from build123d import *

# Parameters (mm, degrees)
ESQUISSE1_W             = 39.8
ESQUISSE1_H             = 4.9
BOSS_EXTRU_1_DEPTH      = 5
ENL_V_MAT_EXTRU_1_REACH = 7
BOSS_EXTRU_2_DEPTH      = 5


with BuildPart() as part:
    # Esquisse1 → Boss.-Extru.1 (new body)
    with BuildSketch(Plane.XY):
        Polygon((100.1, 330.041421356), (128.425692604, 301.715728753), (124.890158698, 298.180194847), (153.033008589, 270.037344955), (156.568542495, 273.572878861), (200.043297184, 230.098124172), (196.507763279, 226.562590266), (211.415404008, 211.654949536), (214.950937914, 215.190483442), (230.1, 200.041421356), (230.1, 159.9), (225.1, 159.9), (225.1, 120.1), (230.1, 120.1), (230.1, 79.9), (225.1, 79.9), (225.1, 40.1), (230.1, 40.1), (230.1, -0.1), (-0.1, -0.1), (-0.1, 50.1), (4.9, 50.1), (4.9, 99.9), (-0.1, 99.9), (-0.1, 150.1), (4.9, 150.1), (4.9, 199.9), (-0.1, 199.9), (-0.1, 250.1), (4.9, 250.1), (4.9, 299.9), (-0.1, 299.9), (-0.1, 350.1), (4.9, 350.1), (4.9, 399.9), (-0.1, 399.9), (-0.1, 450.1), (4.9, 450.1), (4.9, 499.9), (-0.1, 499.9), (-0.1, 550.1), (4.9, 550.1), (4.9, 599.9), (-0.1, 599.9), (-0.1, 650.1), (4.9, 650.1), (4.9, 699.9), (-0.1, 699.9), (-0.1, 750.1), (60.1, 750.1), (60.1, 745.1), (74.9, 745.1), (74.9, 750.1), (100.1, 750.1), (100.1, 699.9), (95.1, 699.9), (95.1, 650.1), (100.1, 650.1), (100.1, 599.9), (95.1, 599.9), (95.1, 550.1), (100.1, 550.1), (100.1, 499.9), (95.1, 499.9), (95.1, 450.1), (100.1, 450.1), (100.1, 399.9), (95.1, 399.9), (95.1, 350.1), (100.1, 350.1), align=None)
        with Locations((145, 232.55)):
            Rectangle(ESQUISSE1_W, ESQUISSE1_H, mode=Mode.SUBTRACT)
    extrude(amount=BOSS_EXTRU_1_DEPTH)

    # Esquisse3 → Enlèv. mat.-Extru.1 (cut, up to next)
    with BuildSketch(Plane.XY.offset(5), mode=Mode.PRIVATE) as enl_v_mat_extru_1_sk1:
        with BuildLine():
            Line((225.1, 156.548997307), (230.1, 156.548997307))
            Line((230.1, 156.548997307), (230.1, 200.041421356))
            Line((230.1, 200.041421356), (185.204076401, 244.937344955))
            Line((185.204076401, 244.937344955), (181.668542495, 241.401811049))
            Line((181.668542495, 241.401811049), (195.810678119, 227.259675426))
            ThreePointArc((195.810678119, 227.259675426), (217.487953251, 194.817340544), (225.1, 156.548997307))
        make_face()
    enl_v_mat_extru_1_tool1 = extrude(enl_v_mat_extru_1_sk1.sketch, amount=-ENL_V_MAT_EXTRU_1_REACH, mode=Mode.PRIVATE) & part.part
    add(enl_v_mat_extru_1_tool1.solids().sort_by_distance((215.811514, 201.214449, 5))[0], mode=Mode.SUBTRACT)

    # Esquisse4 → Boss.-Extru.2 (add)
    with BuildSketch(Plane.XY.offset(5)):
        with BuildLine():
            Line((100.1, 350.1), (100.1, 330.041421356))
            Line((100.1, 330.041421356), (114.28355698, 315.857864376))
            ThreePointArc((114.28355698, 315.857864376), (103.786186359, 331.56828974), (100.1, 350.1))
        make_face()
    extrude(amount=-BOSS_EXTRU_2_DEPTH)


solid = part.part
Geometry: final body of the model. Coordinates: model frame, mm. Coordinates: 2 decimals unless noted, no trailing zeros. Write each loop counter-clockwise with the first axis right and the second up, starting at its lowest first coordinate (ties: lowest second). Pieces come first, ordered by that corner, then holes. Notation, with made-up numbers: (69.25, -3.5) - (92.25, -3.5) arc R29 ccw to (92.25, 24.5) - close; hole circle Ø9 at (2.25, -24). An arc over 180 degrees is marked (long way). Return JSON: item names as keys, results as strings.
Item 1: Pull-direction query (Y, two-part tool) for faces 1 (the face through (188.64, 234.43, 2.54)), 2 (the face through (103.9, 331.3, 2.5)), 3 (the face through (88, 297, 0)); classes: +Y half, -Y half, draft (parallel to the pull), parting line (faces both ways), or undercut.
Completed:
{"face 1": "undercut", "face 2": "+Y half", "face 3": "draft"}
Item 2: Pin query (flat end, axial travel): pin 1 Ø2.5 at (y, z) = (746.5, 2) entering from +X; pin 2 Ø2.5 at (y, z) = (233, 3) entering from +X; pin 3 Ø1.5 at (y, z) = (162.5, 1.5) entering from +X. Return the tip coordinate at first contact, or that it passes through.
Completed:
{"pin 1": "stops at x = 100.1", "pin 2": "stops at x = 191.32", "pin 3": "stops at x = 224.96"}
Item 3: Section query B-B (y = 670). Output: boundary loops of the cut face in (x, z), and give its area (3 significant figures).
Completed:
{"outline": "(4.9, 0) - (95.1, 0) - (95.1, 5) - (4.9, 5) - close", "area": "451 mm2"}
Item 4: Line query: L1, parallel to X at y = 538, z = 2.95; L2, parallel to Y at x = 66.5, z = 3.9; L3, parallel to Y at x = 162.5, z = 3.4. Output: solid intervals per line, ascending.
Completed:
{"L1": "x = -0.1 to 100.1", "L2": "y = -0.1 to 745.1", "L3": "y = -0.1 to 230.1, 235 to 267.64"}
Item 5: Section query A-A (y = 538). Output: boundary loops of the cut face in (x, z), and give its area (3 significant figures).
Completed:
{"outline": "(-0.1, 0) - (100.1, 0) - (100.1, 5) - (-0.1, 5) - close", "area": "501 mm2"}
